The model under review builds one solid part; all positions refer to its coordinate system, in mm. A direction names the side the tool comes from. Round coordinates to 2 decimals unless told otherwise and drop trailing zeros. Order: outer loops, then holes, each group sorted by start corner. A loop starts at its lowest first (then second) coordinate and runs counter-clockwise, first axis right, second up.
```python
from build123d import *

# Parameters (mm, degrees)
SKETCH_1_R          = 28
SKETCH_1_R_2        = 24
EXTRUDE_1_DEPTH     = 5
SKETCH_1_3_R        = 9
EXTRUDE_2_DEPTH     = 10
SKETCH_2_R          = 2.5
CUT_EXTRUDE_1_DEPTH = 41.841155713
SKETCH_3_R          = 2


with BuildPart() as part:
    # 草图1 → 凸台-拉伸1 (new body)
    # profile 1 of 12: a face of its own
    with BuildSketch(Plane.XY):
        Circle(SKETCH_1_R)
        Circle(SKETCH_1_R_2, mode=Mode.SUBTRACT)
    # profile 2 of 12: a face of its own
    with BuildSketch(Plane.XY):
        with BuildLine():
            Line((-11.87931448, 20.853821892), (-6.26655053, 9.838152398))
            Line((-6.26655053, 9.838152398), (-5.392518481, 12.528146446))
            Line((-5.392518481, 12.528146446), (-10.101735892, 21.770506011))
            ThreePointArc((-10.101735892, 21.770506011), (-11.000078241, 21.33068866), (-11.87931448, 20.853821892))
        make_face()
    # profile 3 of 12: a face of its own
    with BuildSketch(Plane.XY):
        with BuildLine():
            ThreePointArc((-8.559508647, 2.781152949), (-6.678325674, 6.033238449), (-3.633390081, 8.233983029))
            Line((-3.633390081, 8.233983029), (1.47456694, 23.95465826))
            ThreePointArc((1.47456694, 23.95465826), (-0.105101651, 23.999769866), (-1.684314548, 23.940824641))
            Line((-1.684314548, 23.940824641), (-5.392518481, 12.528146446))
            Line((-5.392518481, 12.528146446), (-6.26655053, 9.838152398))
            Line((-6.26655053, 9.838152398), (-8.559508647, 2.781152949))
        make_face()
    # profile 4 of 12: a face of its own
    with BuildSketch(Plane.XY):
        with BuildLine():
            Line((16.162253144, 17.742084807), (7.420168337, 9))
            Line((7.420168337, 9), (10.248595461, 9))
            Line((10.248595461, 9), (17.583373541, 16.33477808))
            ThreePointArc((17.583373541, 16.33477808), (16.887479331, 17.053241388), (16.162253144, 17.742084807))
        make_face()
    # profile 5 of 12: a face of its own
    with BuildSketch(Plane.XY):
        with BuildLine():
            Line((7.420168337, 9), (0, 9))
            ThreePointArc((0, 9), (3.674234614, 8.215838363), (6.708203932, 6))
            Line((6.708203932, 6), (23.237900077, 6))
            ThreePointArc((23.237900077, 6), (22.792659325, 7.51629436), (22.248595461, 9))
            Line((22.248595461, 9), (10.248595461, 9))
            Line((10.248595461, 9), (7.420168337, 9))
        make_face()
    # profile 6 of 12: a face of its own
    with BuildSketch(Plane.XY):
        with BuildLine():
            Line((10.852466764, -4.275846499), (8.559508647, 2.781152949))
            ThreePointArc((8.559508647, 2.781152949), (8.889195065, 1.407910185), (9, 0))
            ThreePointArc((9, 0), (8.689464685, -2.34375841), (7.779288115, -4.525779096))
            Line((7.779288115, -4.525779096), (12.887245135, -20.246454327))
            ThreePointArc((12.887245135, -20.246454327), (14.191739808, -19.354444483), (15.434702745, -18.378518742))
            Line((15.434702745, -18.378518742), (11.726498813, -6.965840547))
            Line((11.726498813, -6.965840547), (10.852466764, -4.275846499))
        make_face()
    # profile 7 of 12: a face of its own
    with BuildSketch(Plane.XY):
        with BuildLine():
            Line((21.868136258, -9.888610449), (10.852466764, -4.275846499))
            Line((10.852466764, -4.275846499), (11.726498813, -6.965840547))
            Line((11.726498813, -6.965840547), (20.968858378, -11.675057959))
            ThreePointArc((20.968858378, -11.675057959), (21.437114452, -10.791205863), (21.868136258, -9.888610449))
        make_face()
    # profile 8 of 12: a face of its own
    with BuildSketch(Plane.XY):
        with BuildLine():
            Line((-0.712975015, -11.642618467), (5.290067271, -7.281152949))
            ThreePointArc((5.290067271, -7.281152949), (1.856630381, -8.806413778), (-1.900339469, -8.797085307))
            Line((-1.900339469, -8.797085307), (-15.273144562, -18.512996926))
            ThreePointArc((-15.273144562, -18.512996926), (-14.021681764, -19.477998884), (-12.709424559, -20.358549246))
            Line((-12.709424559, -20.358549246), (-3.001220626, -13.305126218))
            Line((-3.001220626, -13.305126218), (-0.712975015, -11.642618467))
        make_face()
    # profile 9 of 12: a face of its own
    with BuildSketch(Plane.XY):
        with BuildLine():
            ThreePointArc((-4.623906358, -23.550360719), (-3.638613979, -23.722573391), (-2.647001666, -23.853582167))
            Line((-2.647001666, -23.853582167), (-0.712975015, -11.642618467))
            Line((-0.712975015, -11.642618467), (-3.001220626, -13.305126218))
            Line((-3.001220626, -13.305126218), (-4.623906358, -23.550360719))
        make_face()
    # profile 10 of 12: a face of its own
    with BuildSketch(Plane.XY):
        with BuildLine():
            Line((-23.504073256, -4.853714083), (-11.293109556, -2.919687432))
            Line((-11.293109556, -2.919687432), (-13.581355167, -1.257179681))
            Line((-13.581355167, -1.257179681), (-23.826589668, -2.879865413))
            ThreePointArc((-23.826589668, -2.879865413), (-23.685901563, -3.870150793), (-23.504073256, -4.853714083))
        make_face()
    # profile 11 of 12: a face of its own
    with BuildSketch(Plane.XY):
        with BuildLine():
            ThreePointArc((-5.290067271, -7.281152949), (-7.801666869, -4.487091939), (-8.953762497, -0.911118625))
            Line((-8.953762497, -0.911118625), (-22.32656759, 8.804792993))
            ThreePointArc((-22.32656759, 8.804792993), (-22.857615717, 7.31637914), (-23.2895591, 5.796243347))
            Line((-23.2895591, 5.796243347), (-13.581355167, -1.257179681))
            Line((-13.581355167, -1.257179681), (-11.293109556, -2.919687432))
            Line((-11.293109556, -2.919687432), (-5.290067271, -7.281152949))
        make_face()
    # profile 12 of 12: a face of its own
    with BuildSketch(Plane.XY):
        Polygon((7, 0), (3.5, 6.062177826), (-3.5, 6.062177826), (-7, 0), (-3.5, -6.062177826), (3.5, -6.062177826), align=None)
    extrude(amount=EXTRUDE_1_DEPTH)

    # 草图1<3> → 凸台-拉伸2 (add)
    with BuildSketch(Plane.XY):
        with Locations(Location((0, 0, 0), (0, 0, 185.810314896))):
            Circle(SKETCH_1_3_R)
        Polygon((3.5, 6.062177826), (-3.5, 6.062177826), (-7, 0), (-3.5, -6.062177826), (3.5, -6.062177826), (7, 0), align=None, mode=Mode.SUBTRACT)
    extrude(amount=EXTRUDE_2_DEPTH)

    # 草图2 → 切除-拉伸1 (cut, through all)
    with BuildSketch(Plane(origin=(0, 0, 0), x_dir=(-1, 0, 0), z_dir=(0, 0, -1))):
        Circle(SKETCH_2_R)
    extrude(amount=-CUT_EXTRUDE_1_DEPTH, mode=Mode.SUBTRACT)

    # 草图3 → 切除-旋转1 (revolve, cut)
    with BuildSketch(Plane(origin=(0, 0, 0), x_dir=(1, 0, 0), z_dir=(0, 1, 0))):
        with Locations((-28, -2.5)):
            Circle(SKETCH_3_R)
    revolve(axis=Axis((0, 0, 0), (0, 0, 1)), mode=Mode.SUBTRACT)


solid = part.part
```
(1) Consider section A-A (z = 6.75). Write out the cut boundary in (x, y), and give its area (3 significant figures).
Data:
outline: circle Ø18 at (0, 0); hole (-7, 0) - (-3.5, -6.06) - (3.5, -6.06) - (7, 0) - (3.5, 6.06) - (-3.5, 6.06) - close
area: 127 mm2
(2) Draft analysis for pull direction Y (two halves, no side actions). For faces 3 (the flat face through (16.283, -9.287, 2.465)), 4 (the flat face through (-6, -3, 10)), 5 (the flat face through (5.226, -3.074, 7.465)), state which applies: pulls with the +Y half, pulls with the -Y half, needs draft (parallel to the pull), parting line crosses it, or undercut.
Data:
face 3: undercut
face 4: needs draft
face 5: undercut
(3) For faces 1 (the flat face through (-5.226, 3.074, 7.465)), 2 (the flat face through (-1.694, -17.834, 2.465)), list the 3-axis set-ups (+Z, -Z, +X, -X, +Y, -Y) from which the entire face can be reached by the end or side of a thin tool; tool diameter is ignored.
Data:
face 1: +Z
face 2: +Z, -Z
(4) Consider section B-B (y = 1.5). State how many separate pieces and enclosed holes the cut face has, and give its area (3 significant figures).
Data:
separate pieces: 5
enclosed holes: 0
area: 150 mm2
(5) To check wall thickness, follow probe 1 along X at (y, z) = (11, 3.5); probe 2 along Z at (x, y) = (-18, 17.5); probe 3 along X at (y, z) = (-16, 4.75). State the ranges of each line that lie inside material, in increasing order.
Data:
probe 1: x = -23.85 to -21.33, -6.86 to -2.73, 9.42 to 12.25, 21.33 to 23.85
probe 2: z = 0 to 5
probe 3: x = -22.98 to -17.89, -11.81 to -6.71, -3.43 to -1.4, 11.51 to 14.66, 17.89 to 22.98
(6) Insertion check: pin 1 (5 mm diameter, centred on x = 21.5, y = 6, fed in from +Z); pin 2 (1.5 mm diameter, centred on x = 17.5, z = 3, fed in from +Y); pin 3 (10 mm diameter, centred on x = 13, y = 14, fed in from -Z); pin 4 (6 mm diameter, centred on x = -13, z = 4.5, fed in from -Y). Each pin has a flat end and moves straight along its axis. Give the tip position at first contact, or say it passes through.
Data:
pin 1: stops at z = 5
pin 2: stops at y = 20.08
pin 3: stops at z = 0
pin 4: stops at y = -26.15
